Input: part model. Units: mm. Frame: model coordinates. Face numbers are marked on the shaded views. Coordinates: 2 decimals unless noted, no trailing zeros. Loops run counter-clockwise (first coordinate to the right, second up) from the corner with the lowest first, then second, coordinate; pieces in that order, holes last. Notation, with made-up numbers: M 70.5,-36 L 108.5,-36 A20 ccw 108.5,-2 Z; hole C 12,74 d10. An arc over 180 degrees is marked long. Use a Markdown table: item, result. Add a question column.
1. Section A-A on y = 0. State how many separate pieces and enclosed holes the cut face has, then the cut area to 3 significant figures.
2. Pin query (flat end, axial travel): pin 1 (12 mm diameter, centred on x = 0.5, z = -41.5, fed in from -Y); pin 2 (1.5 mm diameter, centred on x = 9, z = -45, fed in from +Y); pin 3 (4 mm diameter, centred on x = 2.5, z = -2.5, fed in from -Y). Return the tip coordinate at first contact, or that it passes through.
3. Line query: L1, parallel to Z at x = -13.1, y = 0; L2, parallel to Z at x = 10.25, y = 0; L3, parallel to Z at x = 13.75, y = 11.5. Output: solid intervals per line, ascending. Write a range as [from, to].
4. Section C-C on x = -5. Output: boundary loops of the cut face in (y, z).
5. Draft query along Z for the marked faces 1, 2 and 3. Return one class per face: +Z half, -Z half, draft (parallel to the pull), parting line (faces both ways), or undercut.
```python
from build123d import *

# Parameters (mm, degrees)
FILLET1_R          = 2
FILLET2_R          = 2
CUT_EXTRUDE2_DEPTH = 2
CIRPATTERN1_COUNT  = 3


with BuildPart() as part:
    # Sketch1 → Revolve2 (revolve)
    with BuildSketch(Plane.XY):
        Polygon((-15, 60), (-7, 60), (-7, 55), (15, 55), (15, 0), (13, 0), (13, 53), (-9, 53), (-9, 58), (-15, 58), align=None)
    revolve(axis=Axis((-15, 0, 0), (1, 0, 0)))

    # Fillet1
    fillet1_edges = [part.edges().sort_by_distance(p)[0] for p in [
        (15, -55, 0),
        (-9, -58, 0),
    ]]
    fillet(fillet1_edges, radius=FILLET1_R)

    # Fillet2
    fillet2_edges = [part.edges().sort_by_distance(p)[0] for p in [
        (-7, -60, 0),
    ]]
    fillet(fillet2_edges, radius=FILLET2_R)

    # Sketch2 → Cut-Extrude2 (cut)
    with BuildSketch(Plane(origin=(15, 0, 0), x_dir=(0, 0, -1), z_dir=(1, 0, 0))):
        with BuildLine():
            Line((-22.627416998, 22.627416998), (-21.213203436, 21.213203436))
            ThreePointArc((-21.213203436, 21.213203436), (0, 30), (21.213203436, 21.213203436))
            Line((21.213203436, 21.213203436), (22.627416998, 22.627416998))
            ThreePointArc((22.627416998, 22.627416998), (0, 32), (-22.627416998, 22.627416998))
        make_face()
        with BuildLine():
            Line((-25.455844123, 25.455844123), (-24.04163056, 24.04163056))
            ThreePointArc((-24.04163056, 24.04163056), (0, 34), (24.04163056, 24.04163056))
            Line((24.04163056, 24.04163056), (25.455844123, 25.455844123))
            ThreePointArc((25.455844123, 25.455844123), (0, 36), (-25.455844123, 25.455844123))
        make_face()
        with BuildLine():
            Line((-28.284271247, 28.284271247), (-26.870057685, 26.870057685))
            ThreePointArc((-26.870057685, 26.870057685), (0, 38), (26.870057685, 26.870057685))
            Line((26.870057685, 26.870057685), (28.284271247, 28.284271247))
            ThreePointArc((28.284271247, 28.284271247), (0, 40), (-28.284271247, 28.284271247))
        make_face()
        with BuildLine():
            Line((-31.112698372, 31.112698372), (-29.69848481, 29.69848481))
            ThreePointArc((-29.69848481, 29.69848481), (0, 42), (29.69848481, 29.69848481))
            Line((29.69848481, 29.69848481), (31.112698372, 31.112698372))
            ThreePointArc((31.112698372, 31.112698372), (0, 44), (-31.112698372, 31.112698372))
        make_face()
        with BuildLine():
            Line((-33.941125497, 33.941125497), (-32.526911935, 32.526911935))
            ThreePointArc((-32.526911935, 32.526911935), (0, 46), (32.526911935, 32.526911935))
            Line((32.526911935, 32.526911935), (33.941125497, 33.941125497))
            ThreePointArc((33.941125497, 33.941125497), (0, 48), (-33.941125497, 33.941125497))
        make_face()
    cut_extrude2 = extrude(amount=-CUT_EXTRUDE2_DEPTH, mode=Mode.SUBTRACT)

    # CirPattern1: Cut-Extrude2 ×3 about axis
    cirpattern1_axis = Axis((0, 0, 0), (1, 0, 0))
    for i in range(1, CIRPATTERN1_COUNT):
        add(cut_extrude2.rotate(cirpattern1_axis, i * 360 / CIRPATTERN1_COUNT), mode=Mode.SUBTRACT)


solid = part.part
```
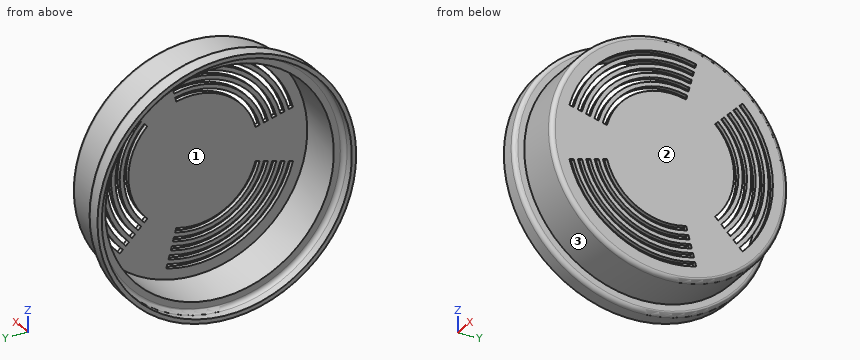
Answers below:
| question | item | result |
|---|---|---|
| 1 | separate pieces | 11 |
| 1 | enclosed holes | 0 |
| 1 | area | 310 mm² |
| 2 | pin 1 | stops at y = -42.01 |
| 2 | pin 2 | stops at y = 32.66 |
| 2 | pin 3 | stops at y = -55 |
| 3 | L1 | z = [-60, -58], [58, 60] |
| 3 | L2 | z = [-55, -53], [53, 55] |
| 3 | L3 | z = [-53.64, -46.6], [-44.54, 44.54], [46.6, 53.64] |
| 4 | outline | C 0,0 d110; hole C 0,0 d106 |
| 5 | face 1 | undercut |
| 5 | face 2 | draft |
| 5 | face 3 | parting line |
